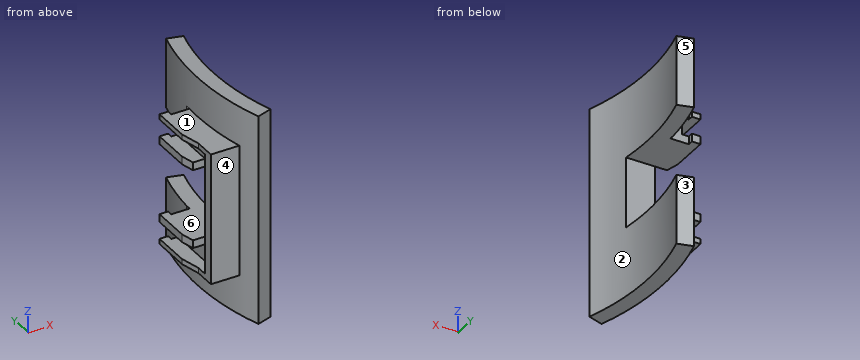
from build123d import *

# Parameters (mm, degrees)
BOSS_EXTRUDE2_DEPTH      = 40
BOSS_EXTRUDE2_DEPTH_BACK = 40
SKETCH5_W                = 50
SKETCH5_H                = 30
BOSS_EXTRUDE1_DEPTH      = 10
BOSS_EXTRUDE1_DEPTH_BACK = 4
SKETCH6_W                = 33
SKETCH6_H                = 6.7
SKETCH6_W_2              = 6.5
SKETCH6_H_2              = 26.2
CUT_EXTRUDE1_DEPTH       = 5.8
CUT_EXTRUDE2_DEPTH       = 50
SKETCH8_W                = 7
SKETCH8_H                = 2
CUT_EXTRUDE3_DEPTH       = 50
SKETCH9_W                = 27
SKETCH9_H                = 14.5
SKETCH9_H_2              = 5
SKETCH9_H_3              = 24.261575761
CUT_EXTRUDE4_DEPTH       = 21.623624402


with BuildPart() as part:
    # Sketch3 → Boss-Extrude2 (new body, two sides)
    with BuildSketch(Plane.XY) as boss_extrude2_sk:
        with BuildLine():
            ThreePointArc((-90.797027671, 24.32899024), (-93.966810921, -2.497688001), (-89.376375598, -29.11809549))
            Line((-89.376375598, -29.11809549), (-95.081250636, -30.97669733))
            ThreePointArc((-95.081250636, -30.97669733), (-99.964692469, -2.657114895), (-96.592582629, 25.88190451))
            Line((-96.592582629, 25.88190451), (-90.797027671, 24.32899024))
        make_face()
    extrude(amount=BOSS_EXTRUDE2_DEPTH)
    extrude(boss_extrude2_sk.sketch, amount=-BOSS_EXTRUDE2_DEPTH_BACK)

    # Sketch5 → Boss-Extrude1 (add, two sides)
    with BuildSketch(Plane.ZY.offset(100)) as boss_extrude1_sk:
        with Locations((0, -7.635182233)):
            Rectangle(SKETCH5_W, SKETCH5_H)
    extrude(amount=BOSS_EXTRUDE1_DEPTH)
    extrude(boss_extrude1_sk.sketch, amount=-BOSS_EXTRUDE1_DEPTH_BACK)

    # Sketch6 → Cut-Extrude1 (cut)
    with BuildSketch(Plane.ZY.offset(110)):
        with Locations((0, -15.485182233)):
            Rectangle(SKETCH6_W, SKETCH6_H)
        with Locations((-19.75, -5.735182233)):
            Rectangle(SKETCH6_W_2, SKETCH6_H_2)
        with Locations((19.75, -5.735182233)):
            Rectangle(SKETCH6_W_2, SKETCH6_H_2)
    extrude(amount=-CUT_EXTRUDE1_DEPTH, mode=Mode.SUBTRACT)

    # Sketch7 → Cut-Extrude2 (cut)
    with BuildSketch(Plane(origin=(0, 0, -25), x_dir=(-1, 0, 0), z_dir=(0, 0, -1))):
        Polygon((108.2, -22.635182233), (108.2, -14.635182233), (110, -7.135182233), (110, -22.635182233), align=None)
    extrude(amount=-CUT_EXTRUDE2_DEPTH, mode=Mode.SUBTRACT)

    # Sketch8 → Cut-Extrude3 (cut)
    with BuildSketch(Plane(origin=(0, 0, -25), x_dir=(-1, 0, 0), z_dir=(0, 0, -1))):
        with Locations((103.228428541, 6.364817767)):
            Rectangle(SKETCH8_W, SKETCH8_H)
    extrude(amount=-CUT_EXTRUDE3_DEPTH, mode=Mode.SUBTRACT)

    # Sketch9 → Cut-Extrude4 (cut, through all)
    with BuildSketch(Plane.ZY.offset(110)):
        with Locations((0, 0.114817767)):
            Rectangle(SKETCH9_W, SKETCH9_H)
        with Locations((0, -9.635182233)):
            Rectangle(SKETCH9_W, SKETCH9_H_2)
        with Locations((0, 19.495605647)):
            Rectangle(SKETCH9_W, SKETCH9_H_3)
    extrude(amount=-CUT_EXTRUDE4_DEPTH, mode=Mode.SUBTRACT)


solid = part.part
Source: CAD feature listing. Evaluate the final solid. Frame: model axes, mm. Face numbers are marked on the shaded views. A direction names the side the tool comes from. Give positions to 0.01 mm unless a question says otherwise; leave off trailing zeros. Write each loop counter-clockwise with the first axis right and the second up, starting at its lowest first coordinate (ties: lowest second). Pieces come first, ordered by that corner, then holes. Notation, with made-up numbers: (-3.5, 56.5) -> (18.5, 56.5) arc R25 ccw to (18.5, 75.5) -> close; hole circle Ø11 at (75, 28). An arc over 180 degrees is marked (long way). Write item = value, one per line.
Q1. Cut plane C-C on x = -101.25. Return loops of the section in (y, z), then the cut area to 4 significant figures.
Here are the results:
outline = (-22.64, -25) -> (5.36, -25) -> (5.36, -13.5) -> (-12.14, -13.5) -> (-12.14, 13.5) -> (5.36, 13.5) -> (5.36, 25) -> (-22.64, 25) -> close
area = 927.5 mm²
Q2. Cut plane B-B on y = -11. Return loops of the section in (x, z), then the cut area to 3 significant figures.
Here are the results:
outline = (-109.07, -25) -> (-99.39, -25) -> (-99.39, -40) -> (-93.35, -40) -> (-93.35, -13.5) -> (-109.07, -13.5) -> (-109.07, -16.5) -> (-104.2, -16.5) -> (-104.2, -23) -> (-109.07, -23) -> close; (-109.07, 13.5) -> (-93.35, 13.5) -> (-93.35, 40) -> (-99.39, 40) -> (-99.39, 25) -> (-109.07, 25) -> (-109.07, 23) -> (-104.2, 23) -> (-104.2, 16.5) -> (-109.07, 16.5) -> close
area = 479 mm²
Q3. Mould query, pull axis Y, two halves, no side actions, for the marked faces 1, 2 and 3. Classes: +Y half, -Y half, draft (parallel to the pull), parting line (faces both ways), or undercut.
Here are the results:
face_1 = draft
face_2 = undercut
face_3 = +Y half
Q4. Cut plane D-D on y = 16. Return loops of the section in (x, z).
Here are the results:
outline = (-98.71, -40) -> (-92.63, -40) -> (-92.63, -13.5) -> (-98.71, -13.5) -> close; (-98.71, 13.5) -> (-92.63, 13.5) -> (-92.63, 40) -> (-98.71, 40) -> close
Q5. Cut plane A-A on z = 22. Return loops of the section in (x, y).
Here are the results:
outline = (-108.2, -22.64) -> (-97.4, -22.64) arc R100 ccw to (-95.08, -30.98) -> (-89.38, -29.12) arc R94 cw to (-90.8, 24.33) -> (-96.59, 25.88) arc R100 ccw to (-99.73, 7.36) -> (-99.73, 5.36) -> (-104.2, 5.36) -> (-104.2, -18.84) -> (-108.2, -18.84) -> close
Q6. Reachability of the marked faces 4, 5 and 6 from +Z, -Z, +X, -X, +Y, -Y: full face, straight path, thin tool, end or side. Return the list, or none.
Here are the results:
face_4 = +Z, -Z, -X, -Y
face_5 = +Z, -Z, +X, +Y
face_6 = +X, -X, +Y
Q7. Line query: line 1 (Z direction, x = -108.75, y = 5); line 2 (Z direction, x = -94.25, y = 3); line 3 (Y direction, x = -99.5, z = 11). Output: solid intervals per line, ascending. Write a range as from..to.
Here are the results:
line_1 = -25..-23, -16.5..-13.5, 13.5..16.5, 23..25
line_2 = -40..-13.5, 13.5..40
line_3 = -22.64..-12.14
Q8. First-contact query: pin 1 (0.9 mm diameter, centred on x = -106, z = 15.5, fed in from -Y); pin 2 (0.6 mm diameter, centred on y = 6.5, z = -24.5, fed in from +X); pin 3 (1.5 mm diameter, centred on x = -91.5, z = -7.5, fed in from -Y). Flat tips, straight axial feed; report the tip coordinate or a pass-through.
Here are the results:
pin_1 = -22.64
pin_2 = -93.75
pin_3 = -30.05
